Geometry check sheet. Reference: the model listing, model coordinates, mm. Round coordinates to 2 decimals unless told otherwise and drop trailing zeros. Order: outer loops, then holes, each group sorted by start corner. A loop starts at its lowest first (then second) coordinate and runs counter-clockwise, first axis right, second up. Notation, with made-up numbers: (51.25, 26.25) - (91.25, 26.25) arc R21 ccw to (91.25, 31.25) - close; hole circle Ø9 at (-29.5, 37.5). An arc over 180 degrees is marked (long way). Use a Markdown table: item, result. Add a question column.
(1) Gauge pin test, flat ends, axial feed: P1, Ø3, axis at x = -4.5, z = 7.5, coming from the +Y side; P2, Ø6, axis at y = 41, z = 21.5, coming from the +X side; P3, Ø6, axis at y = 37.5, z = 8.5, coming from the -X side; P4, Ø2.5, axis at y = -2, z = 11, coming from the -X side. Record the tip position at first contact, or that the pin passes through.
(2) Thickness scan on line 1 along X through (y, z) = (-1, 23.25); line 2 along X through (y, z) = (7.5, 3); line 3 along Y through (x, z) = (-3, 7.5). Record the ranges inside material, lowest first. Write a range as [from, to].
(3) Section check B-B on x = 0.75. Record the boundary of the cut face in (y, z).
(4) Section check C-C on y = 38. Record the boundary of the cut face in (x, z).
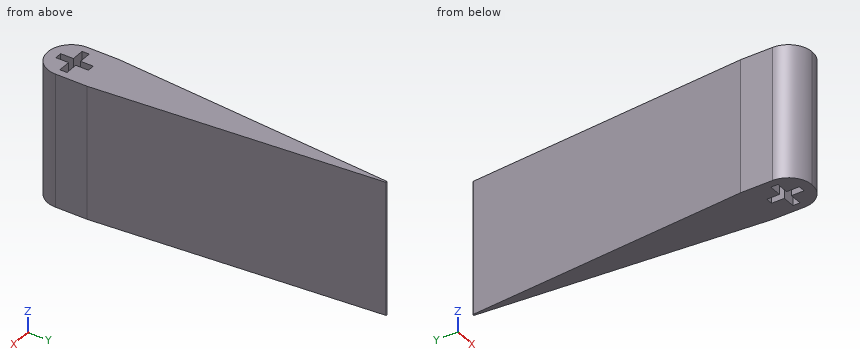
Autodesk Inventor part; units mm, degrees
ref_plane "YZ Plane" through (0, 0, 0) normal (1, 0, 0) x (0, 1, 0)
ref_plane "XZ Plane" through (0, 0, 0) normal (0, 1, 0) x (-1, 0, 0)
ref_plane "XY Plane" through (0, 0, 0) normal (0, 0, 1) x (1, 0, 0)
sketch "Sketch1" plane through (0, 0, 0) normal (0, 0, 1) x (1, 0, 0)
  line L0 (-7.5832, 61.4886) -> (1.4084, 61.4886)
  line L1 (1.4084, 61.4886) -> (1.4084, -4.9324)
  line L2 (1.4084, -4.9324) -> (-7.5832, -4.9324)
  line L3 (-7.5832, -4.9324) -> (-7.5832, 61.4886)
  point P0 (0, 0)
  dimension "d0" = 8.9916
  dimension "d1" = 66.421
extrude "Extrusion1" add sketch "Sketch1" along normal blind 25.4
sketch "Sketch2" plane through (0, 0, 25.4) normal (0, 0, 1) x (1, 0, 0)
  line L0 (-7.5832, -4.9324) -> (1.4084, -4.9324)
  line L1 (-3.0874, -4.9324) -> (-3.0874, 0.1476) construction
  circle A0 centre (-3.0874, 0.1476) radius 3.175 construction
  line L2 (-3.0874, 0.1476) -> (-3.7626, 3.25) construction
  line L3 (-3.0874, 0.1476) -> (-2.4123, 3.25) construction
  line L4 (-3.7626, 3.25) -> (-2.4123, 3.25)
  line L5 (-3.0874, 0.1476) -> (-6.1898, -0.5275) construction
  line L6 (-6.1898, -0.5275) -> (-6.1898, 0.8228)
  line L7 (-3.0874, 0.1476) -> (-2.4123, -2.9547) construction
  line L8 (-2.4123, -2.9547) -> (-3.7626, -2.9547)
  line L9 (-3.0874, 0.1476) -> (0.0149, 0.8228) construction
  line L10 (0.0149, 0.8228) -> (0.0149, -0.5275)
  line L11 (-3.7626, 3.25) -> (-3.7626, 0.8228)
  line L12 (-3.7626, -0.5275) -> (-3.7626, -2.9547)
  line L13 (-6.1898, -0.5275) -> (-3.7626, -0.5275)
  line L14 (-2.4123, -0.5275) -> (0.0149, -0.5275)
  line L15 (-2.4123, -2.9547) -> (-2.4123, -0.5275)
  line L16 (-2.4123, 0.8228) -> (-2.4123, 3.25)
  line L17 (-2.4123, 0.8228) -> (0.0149, 0.8228)
  line L18 (-6.1898, 0.8228) -> (-3.7626, 0.8228)
  point P0 (0, 0)
  dimension "d4" = 5.08
  dimension "d5" = 6.35
  dimension "d18" = 360
fillet "Fillet1" radius 4.4958 2 edges at (1.4084, -4.9324, 12.7) (-7.5832, -4.9324, 12.7)
chamfer "Chamfer1" distance 4.4958 distance2 55.88 1 edges at (-7.5832, 61.4886, 12.7) measured on face at (-1.5888, 61.4886, 8.4667)
chamfer "Chamfer2" distance 55.88 distance2 4.4958 1 edges at (1.4084, 61.4886, 12.7) measured on face at (1.4084, 20.2051, 8.4667)
sketch "Sketch3" plane through (0, 0, 25.4) normal (0, 0, 1) x (1, 0, 0)
  point P0 (0, 0)
fillet "Fillet2" radius 0.1588 2 edges at (-3.0873, 61.4886, 12.7) (-3.0874, 61.4886, 12.7)
extrude "Extrusion3" cut sketch "Sketch2" against normal blind 25.4
sketch "Sketch4" plane through (0, 0, 25.4) normal (0, 0, 1) x (1, 0, 0)
  line L0 (-6.1898, 0.8228) -> (-6.1898, -0.5275)
  line L1 (-6.1898, 0.1476) -> (-2.5733, 0.1476) construction
  circle A0 centre (-3.0874, 0.1476) radius 0.9548
  point P0 (0, 0)
properties part number "Bistable Flipper"
Check sheet entries:
| question | item | result |
|---|---|---|
| 1 | P1 | stops at y = 59.67 |
| 1 | P2 | stops at x = -1.2 |
| 1 | P3 | stops at x = -5.26 |
| 1 | P4 | stops at x = -7.57 |
| 2 | line 1 | x = [-7.55, -3.76], [-2.41, 1.37] |
| 2 | line 2 | x = [-7.43, 1.26] |
| 2 | line 3 | y = [-4.93, -2.95], [3.25, 59.64] |
| 3 | outline | (-2.78, 0) - (13.79, 0) - (13.79, 25.4) - (-2.78, 25.4) - close |
| 4 | outline | (-4.98, 0) - (-1.2, 0) - (-1.2, 25.4) - (-4.98, 25.4) - close |
